Can you work these out from the model? Positions are in its coordinate system, mm. A direction names the side the tool comes from. Coordinates: 2 decimals unless noted, no trailing zeros. Write each loop counter-clockwise with the first axis right and the second up, starting at its lowest first coordinate (ties: lowest second). Pieces come first, ordered by that corner, then holes. Notation, with made-up numbers: (65, 49.25) -> (78, 49.25) arc R6 cw to (78, 55.25) -> close; hole circle Ø4 at (-33, -25.75). An arc over 180 degrees is marked (long way). Use one line per item in the form item = value.
```python
from build123d import *

# Parameters (mm, degrees)
F2_SIZE2 = 10
F2_SIZE  = 10
F3_SIZE2 = 9.99999
F3_SIZE  = 9.99999
F4_SIZE2 = 3
F4_SIZE  = 3


# Not quite as in the source:
# - a fillet or chamfer is up to 0.001 mm smaller than in the source, because OpenCascade refuses the exact size


with BuildPart() as f1:
    # F0 (on Top) → F1 (revolve)
    with BuildSketch(Plane.XY):
        Polygon((-80, 7.5), (-80, 0), (80, 0), (80, 40), (70, 40), (70, 20), (-55, 20), (-55, 7.5), align=None)
    revolve(axis=Axis((0, 0, 0), (-1, 0, 0)))

    # F2
    f2_edges = [f1.edges().sort_by_distance(p)[0] for p in [
        (70, -20, 0),
    ]]
    chamfer(f2_edges, length=F2_SIZE, length2=F2_SIZE2)

    # F3 (size 10 and 10 in the source; OpenCascade refuses exactly that, so slightly less here)
    f3_edges = [f1.edges().sort_by_distance(p)[0] for p in [
        (80, -40, 0),
    ]]
    chamfer(f3_edges, length=F3_SIZE, length2=F3_SIZE2)

    # F4
    f4_edges = [f1.edges().sort_by_distance(p)[0] for p in [
        (-55, -20, 0),
    ]]
    chamfer(f4_edges, length=F4_SIZE, length2=F4_SIZE2)


solid = f1.part
```
Q1. For faces 1 (the flat face through (-55, 7, 4)), 2 (the flat face through (-80, 0, 0)), which set-ups out of +Z, -Z, +X, -X, +Y, -Y let a thin tool reach every point of the face, with its end or its side?
Return value:
face_1 = -X
face_2 = +Z, -Z, -X, +Y, -Y
Q2. Suppose I cut it at C-C (x = 37.5). Write out the boundary of the cut face in (y, z), then the cut area to 3 significant figures.
Return value:
outline = circle Ø40 at (0, 0)
area = 1,260 mm2
Q3. Will these pins go through, and if not, where does the flat tip stop? pin 1 (8 mm diameter, centred on y = 8.5, z = -8, fed in from -X); pin 2 (4 mm diameter, centred on y = -25, z = 4, fed in from -X); pin 3 (5 mm diameter, centred on y = -4.5, z = 32, fed in from -X).
Return value:
pin_1 = -55
pin_2 = 63.32
pin_3 = 69.81
Q4. If I drill on line 1 (X direction, y = 4, z = 15); line 2 (Z direction, x = 6, y = 3.5); line 3 (Y direction, x = -23.5, z = 8), over which ranges is the centre line in solid material (lowest first)? Write a range as from..to.
Return value:
line_1 = -55..80
line_2 = -19.69..19.69
line_3 = -18.33..18.33
